CAD build for the part. Positions are in the model's coordinates, mm. A direction names the side the tool comes from. Give positions to 0.01 mm unless a question says otherwise; leave off trailing zeros. Write each loop counter-clockwise with the first axis right and the second up, starting at its lowest first coordinate (ties: lowest second). Pieces come first, ordered by that corner, then holes. Notation, with made-up numbers: (45, 34) -> (68, 34) arc R18 ccw to (68, 41) -> close; hole circle Ø5 at (-14, -34.5). An arc over 180 degrees is marked (long way). Answer as a JSON object with one key per item and string values.
```python
from build123d import *


with BuildPart() as part:
    # Çizim1 → Döndür1 (revolve)
    with BuildSketch(Plane(origin=(0, 0, 0), x_dir=(0, 0, -1), z_dir=(1, 0, 0)), mode=Mode.PRIVATE) as d_nd_r1_sk:
        Polygon((7.365702479, 5.625), (27.365702479, 5.625), (27.365702479, 1.875), (-3.884297521, 1.875), (-3.884297521, 5.625), (4.865702479, 5.625), (4.865702479, 7.5), (7.365702479, 7.5), align=None)
    revolve(d_nd_r1_sk.sketch.rotate(Axis((0, 0, 4.380165289), (0, 0, -1)), 90), axis=Axis((0, 0, 4.380165289), (0, 0, -1)))


solid = part.part
```
1) Slice it at C-C (z = -22). List the corners of the cut face in (x, y) (3 decimals), then the cut area to 3 significant figures.
Model answer:
{"outline": "circle Ø11.25 at (0, 0); hole circle Ø3.75 at (0, 0)", "area": "88.4 mm2"}
2) Wall check: probe 1 along Y at (x, z) = (0, -5) (3 decimals); probe 2 along Y at (x, z) = (0, -2.5) (3 decimals); probe 3 along Z at (x, y) = (-5.25, 5.25). Give the ranges that are in metal, low to high.
Model answer:
{"probe 1": "y = -7.5 to -1.875, 1.875 to 7.5", "probe 2": "y = -5.625 to -1.875, 1.875 to 5.625", "probe 3": "z = -7.37 to -4.87"}
3) Mould opens along Y. For faces 4 (the cylindrical face through (4.032, -6.324, -6.133)), 5 (the cylindrical face through (1.01, -1.58, -11.52)), 6 (the flat face through (0.1, 2.4, 3.884)) say: released by +Y, released by -Y, zero draft, split by the parting line, or undercut.
Model answer:
{"face 4": "split by the parting line", "face 5": "undercut", "face 6": "zero draft"}
4) 3-axis set-ups, long thin cutter, end or side, ignore diameter. For faces 1 (the cylindrical face through (2.6, 4.99, -17.51)), 2 (the flat face through (-0.1, 2.4, -27.366)), 3 (the cylindrical face through (2.6, 4.99, -0.55)): which of +Z, -Z, +X, -X, +Y, -Y reach the whole face in a straight line?
Model answer:
{"face 1": "-Z", "face 2": "-Z, +X, -X, +Y, -Y", "face 3": "+Z"}
5) Slice it at D-D (x = -4.25). List the corners of the cut face in (y, z), then the cut area to 3 significant figures.
Model answer:
{"outline": "(-6.18, -7.37) -> (-3.68, -7.37) -> (-3.68, -27.37) -> (3.68, -27.37) -> (3.68, -7.37) -> (6.18, -7.37) -> (6.18, -4.87) -> (3.68, -4.87) -> (3.68, 3.88) -> (-3.68, 3.88) -> (-3.68, -4.87) -> (-6.18, -4.87) -> close", "area": "243 mm2"}
6) Pin check, flat tips, straight feed: pin 1 (3.5 mm diameter, centred on x = 0, y = 0, fed in from +Z); pin 2 (6 mm diameter, centred on y = -4.5, z = -3.5, fed in from -X); pin 3 (6 mm diameter, centred on y = -4, z = -5.5, fed in from -X); pin 4 (2 mm diameter, centred on y = 5, z = -5, fed in from +X). Stop position of each tip, or through.
Model answer:
{"pin 1": "passes through", "pin 2": "stops at x = -7.27", "pin 3": "stops at x = -7.43", "pin 4": "stops at x = 6.34"}
7) Slice it at A-A (y = 0). List the corners of the cut face in (x, z) (3 decimals), then the cut area to 3 significant figures.
Model answer:
{"outline": "(-7.5, -7.366) -> (-5.625, -7.366) -> (-5.625, -27.366) -> (-1.875, -27.366) -> (-1.875, 3.884) -> (-5.625, 3.884) -> (-5.625, -4.866) -> (-7.5, -4.866) -> close; (1.875, -27.366) -> (5.625, -27.366) -> (5.625, -7.366) -> (7.5, -7.366) -> (7.5, -4.866) -> (5.625, -4.866) -> (5.625, 3.884) -> (1.875, 3.884) -> close", "area": "244 mm2"}
